Drawing for the job (mm, zero at the part's lowest x, y, z). A direction names the side the tool comes from. Round coordinates to 2 decimals unless told otherwise and drop trailing zeros. Write each loop counter-clockwise with the first axis right and the second up, starting at its lowest first coordinate (ties: lowest second). Pieces come first, ordered by that corner, then holes. Notation, with made-up numbers: M 6,25 L 33,25 A36 ccw 33,60 Z; hole C 44.25,-2 d2. An arc over 180 degrees is marked long. Use a Markdown table: item, result. Add a question column.
1) Wall check: probe 1 along Z at (x, y) = (13.5, 4.1); probe 2 along X at (y, z) = (3.4, 27); probe 3 along Z at (x, y) = (7.5, 9.25). Give the ranges that are in metal, low to high.
2) Slice it at C-C on y = 1.5. Write the cut outline in (x, z).
3) Slice it at D-D on x = 24. Write the cut outline in (y, z), plus the area to 3 significant figures.
4) Slice it at B-B on y = 15.25. Write the cut outline in (x, z), plus the area to 3 significant figures.
5) Slice it at A-A on z = 27. Write the cut outline in (x, y).
6) Two-plate mould, pull along Z, no slides. Class the marked faces 1, 2 and 3: released by +Z, released by -Z, zero draft, split by the parting line, or undercut.
7) Drop flat-ended pins along their axis: P1, Ø13.5, axis at x = 13, z = 7, coming from the -Y side; P2, Ø1.4, axis at y = 3.5, z = 28.5, coming from the -X side; P3, Ø10, axis at x = 12, y = 14, coming from the -Z side. Give the stop position or say it passes through.
8) Which spindle directions (+Z, -Z, +X, -X, +Y, -Y) get a long thin tool onto all of the face, cutting with end or side? Do the marked faces 4, 5 and 6. Say none if no direction does.
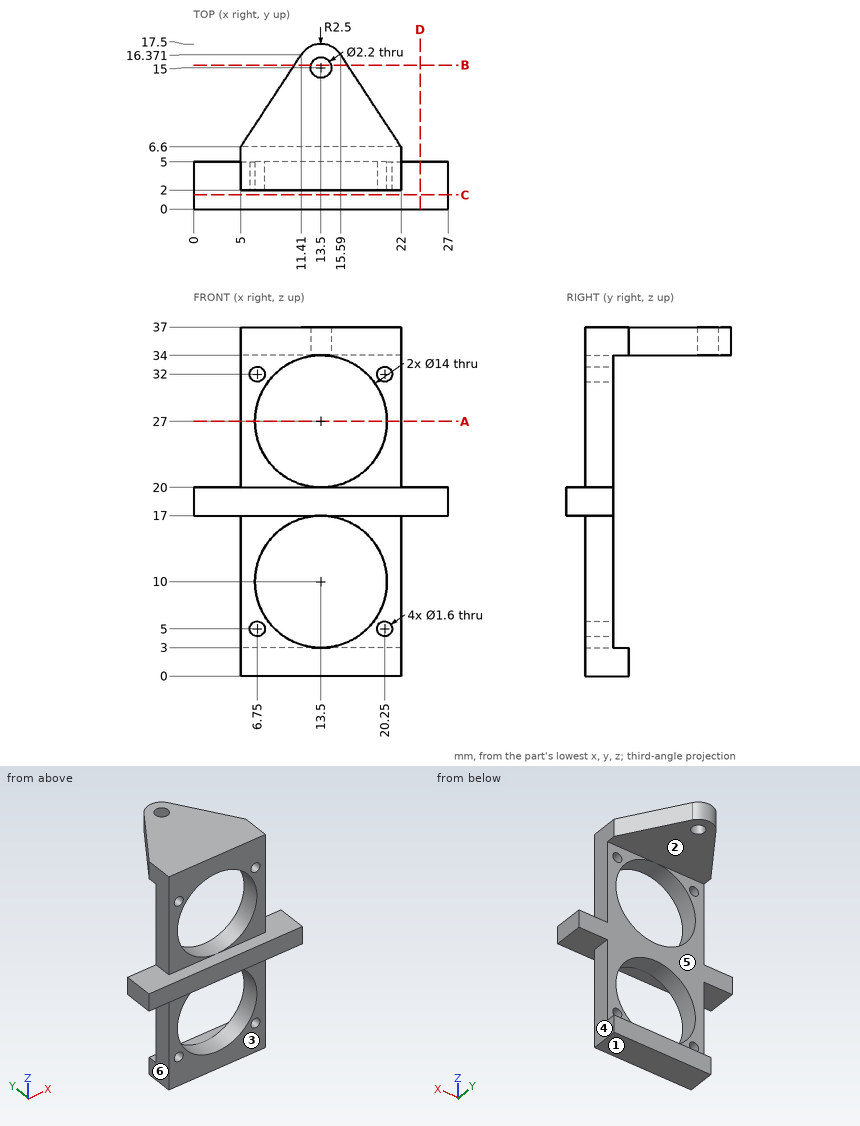
Entries:
| question | item | result |
|---|---|---|
| 1 | probe 1 | z = 0 to 3, 17 to 20, 34 to 37 |
| 1 | probe 2 | x = 5 to 6.5, 20.5 to 22 |
| 1 | probe 3 | z = 34 to 37 |
| 2 | outline | M 0,17 L 27,17 L 27,20 L 0,20 Z |
| 3 | outline | M 0,17 L 5,17 L 5,20 L 0,20 Z |
| 3 | area | 15.0 mm^2 |
| 4 | outline | M 10.67,34 L 12.43,34 L 12.43,37 L 10.67,37 Z; M 14.57,34 L 16.33,34 L 16.33,37 L 14.57,37 Z |
| 4 | area | 10.5 mm^2 |
| 5 | outline | M 5,2 L 6.5,2 L 6.5,5 L 5,5 Z; M 20.5,2 L 22,2 L 22,5 L 20.5,5 Z |
| 6 | face 1 | released by -Z |
| 6 | face 2 | undercut |
| 6 | face 3 | zero draft |
| 7 | P1 | stops at y = 2 |
| 7 | P2 | stops at x = 5 |
| 7 | P3 | stops at z = 34 |
| 8 | face 4 | -Z, +X, +Y, -Y |
| 8 | face 5 | +X, -X, +Y |
| 8 | face 6 | -Z, -X, +Y, -Y |
